The listing builds one solid part. Answer for the finished solid, in the listing's coordinates (mm). Face numbers are marked on the shaded views. Round coordinates to 2 decimals unless told otherwise and drop trailing zeros. Loops run counter-clockwise (first coordinate to the right, second up) from the corner with the lowest first, then second, coordinate; pieces in that order, holes last. Notation, with made-up numbers: M 10.25,-2.75 L 31.25,-2.75 A11 cw 31.25,1.25 Z; hole C -17.5,73.5 d1. An arc over 180 degrees is marked long. Answer as a JSON object with one key per item and string values.
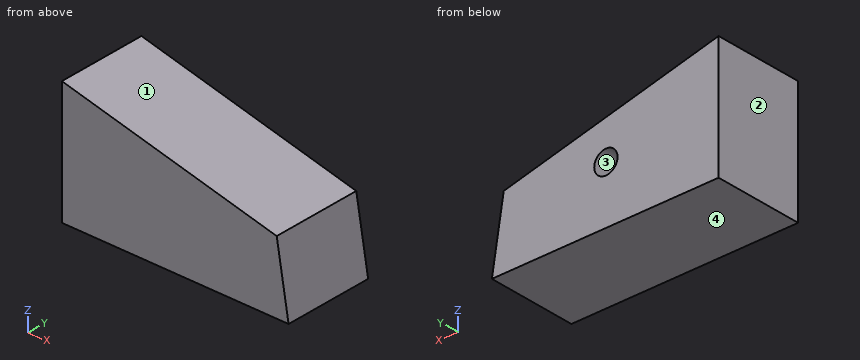
```python
from build123d import *

# Parameters (mm, degrees)
F1_DEPTH = 25.4
F3_D     = 6.6
F3_DEPTH = 12.7
F3_TIP   = 1.9828400428


with BuildPart() as f1:
    # F0 (on Front) → F1 (new body)
    with BuildSketch(Plane.XZ):
        Polygon((-3.3652072307, 20.2556531876), (-64.2102658749, 34.7338579595), (-64.2102658749, 0), (0, 0), align=None)
    extrude(amount=F1_DEPTH)

    # F3
    with Locations(Plane(origin=(0, 0, 0), x_dir=(-1, 0, 0), z_dir=(0, 1, 0))):
        with Locations((32.2950705886, 16.1637682468)):
            Hole(F3_D / 2, depth=F3_DEPTH)
            with Locations((0, 0, -(F3_DEPTH + F3_TIP / 2))):  # 118° drill point
                Cone(0, F3_D / 2, F3_TIP, mode=Mode.SUBTRACT)


solid = f1.part
```
Item 1: The part is cut by section A-A (y = -9.25). Give the vertices of the cut face in (x, z), then the cut area to 3 significant figures.
Values follow:
{"outline": "M -64.21,0 L 0,0 L -3.37,20.26 L -64.21,34.73 Z; hole C -32.3,16.16 d6.6", "area": "1,670 mm^2"}
Item 2: The part is cut by section B-B (x = -54.5). Give the vertices of the cut face in (y, z), then the cut area to 3 significant figures.
Values follow:
{"outline": "M -25.4,0 L 0,0 L 0,32.42 L -25.4,32.42 Z", "area": "824 mm^2"}
Item 3: The part is cut by section C-C (y = -21). Give the vertices of the cut face in (x, z), then the cut area to 3 significant figures.
Values follow:
{"outline": "M -64.21,0 L 0,0 L -3.37,20.26 L -64.21,34.73 Z", "area": "1,710 mm^2"}
Item 4: Flat-ended cylindrical pins translate along their axes: P1, Ø1, axis at x = -57.5, y = -7.5, coming from the +Z side; P2, Ø12, axis at x = -18, y = -20, coming from the +Z side; P3, Ø1.5, axis at x = -38, y = -16.5, coming from the +Z side. Find the tip coordinate at first contact, or state that the pin passes through.
Values follow:
{"P1": "z = 33.26", "P2": "z = 25.17", "P3": "z = 28.68"}
Item 5: Determine the mould class of the marked faces 1, 2, 3 and 4 for opening direction Z: released by +Z, released by -Z, zero draft, split by the parting line, or undercut.
Values follow:
{"face 1": "released by +Z", "face 2": "zero draft", "face 3": "undercut", "face 4": "released by -Z"}
Item 6: Straight lines are drawn through the part: line 1 (Z direction, x = -34, y = -3.5); line 2 (X direction, y = -11.75, z = 6); line 3 (X direction, y = -14.75, z = 2.5). For each, find the intervals that lie inside material, in ascending order.
Values follow:
{"line 1": "0 to 13.34, 18.99 to 27.55", "line 2": "-64.21 to -1", "line 3": "-64.21 to -0.42"}
